Design review of the part built by this model. Coordinates are the model's own, in mm. Round coordinates to 2 decimals unless told otherwise and drop trailing zeros. Order: outer loops, then holes, each group sorted by start corner. A loop starts at its lowest first (then second) coordinate and runs counter-clockwise, first axis right, second up. Notation, with made-up numbers: M 88,1.25 L 117,1.25 A17 ccw 117,10.25 Z; hole C -30,-11 d3. An arc over 180 degrees is marked long. Use a Markdown table: item, result. Add a question column.
(1) To check wall thickness, follow probe 1 along X at (y, z) = (3.5, 1.3); probe 2 along X at (y, z) = (3, 1.85); probe 3 along X at (y, z) = (3.25, 1.5). State the ranges of each line that lie inside material, in increasing order. Write a range as from..to.
(2) For pin 1 (4.5 mm diameter, centred on x = 26.8, y = 5.05, fed in from +Z); pin 2 (3 mm diameter, centred on x = 27.5, y = 11, fed in from +Z), all flat-tipped, find the tip position at first contact; note any pin that passes through.
(3) Take a section at A-A (y = 5.75). Count the separate pieces of the cut face and the enclosed holes in it, then the cut area to 3 significant figures.
(4) Take a section at B-B (x = 3). Write out the cut boundary in (y, z).
```python
from build123d import *

# Parameters (mm, degrees)
ESQUISSE1_R        = 2
BOSS_EXTRU_1_DEPTH = 2
CONG_1_R           = 1
CONG_2_R           = 101


with BuildPart() as part:
    # Esquisse1 → Boss.-Extru.1 (new body)
    with BuildSketch(Plane.XY):
        with BuildLine():
            ThreePointArc((6.353742359, 13.587860686), (-7.923021794, 12.736786316), (-14.996867452, 0.306539744))
            Line((-14.996867452, 0.306539744), (-11.992657898, 0.419710068))
            ThreePointArc((-11.992657898, 0.419710068), (0.419710068, 11.992657898), (11.992657898, -0.419710068))
            Line((11.992657898, -0.419710068), (14.999728999, -0.090166274))
            add(Edge.make_bspline(
                [(6.353742359, 13.587860686), (53.739631024, 4.255841601), (14.999728999, -0.090166274)],
                knots=[0, 0, 0, 1, 1, 1], degree=2))
        make_face()
        with Locations((26.803607687, 5.048670414)):
            Circle(ESQUISSE1_R, mode=Mode.SUBTRACT)
    extrude(amount=BOSS_EXTRU_1_DEPTH)

    # Congé1
    cong_1_edges = [part.edges().sort_by_distance(p)[0] for p in [
        (11.992657898, -0.419710068, 1),
        (-11.992657898, 0.419710068, 1),
        (-14.996867452, 0.306539744, 1),
    ]]
    fillet(cong_1_edges, radius=CONG_1_R)

    # Congé2
    cong_2_edges = [part.edges().sort_by_distance(p)[0] for p in [
        (6.353742359, 13.587860686, 1),
    ]]
    fillet(cong_2_edges, radius=CONG_2_R)


solid = part.part
```
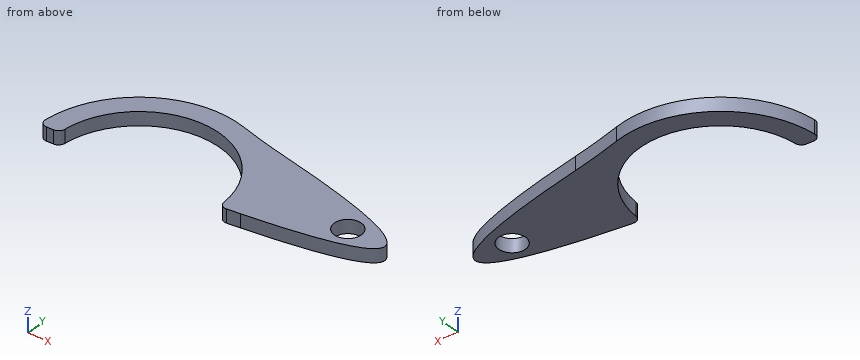
Verdict:
| question | item | result |
|---|---|---|
| 1 | probe 1 | x = -14.59..-11.48, 11.48..25.54, 28.07..31.48 |
| 1 | probe 2 | x = -14.7..-11.62, 11.62..30.57 |
| 1 | probe 3 | x = -14.64..-11.55, 11.55..25.93, 27.68..31.06 |
| 2 | pin 1 | stops at z = 2 |
| 2 | pin 2 | passes through |
| 3 | separate pieces | 3 |
| 3 | enclosed holes | 0 |
| 3 | area | 42.1 mm^2 |
| 4 | outline | M 11.62,0 L 14.7,0 L 14.7,2 L 11.62,2 Z |
